Input: part model. Units: mm. Frame: model coordinates. Face numbers are marked on the shaded views. A direction names the side the tool comes from. Round coordinates to 2 decimals unless told otherwise and drop trailing zeros. Loops run counter-clockwise (first coordinate to the right, second up) from the corner with the lowest first, then second, coordinate; pieces in that order, holes last. Notation, with made-up numbers: (-36, -8) -> (-20, -8) arc R22 ccw to (-20, 29) -> close; hole circle Ø9 at (-3, 86.5). An arc over 180 degrees is marked (long way). One line per question, with ' | ' between items. Start each with the question number.
Q1. Mould query, pull axis X, two halves, no side actions, for the marked faces 1, 2 and 3. Classes: pulls with the +X half, pulls with the -X half, needs draft (parallel to the pull), parting line crosses it, or undercut.
Q2. Cut plane D-D on y = 46.5. Return loops of the section in (x, z), and give its area (3 significant figures).
Q3. Access query for the marked faces 4 and 5. Directions: +Z, -Z, +X, -X, +Y, -Y. A direction counts if a zero-diameter tool reaches every point of the face in a straight line with its end or side. Return the directions, or none.
Q4. Material intervals for L1, parallel to Y at x = 0, z = -2.85; L2, parallel to X at y = 46.5, z = -1; L3, parallel to X at y = 5, z = -1, sorted ascending.
Q5. Cut plane B-B on y = 3.5. Return loops of the section in (x, z).
Q6. Contact query for flat-ended pins moving along their axis: P1, Ø4, axis at x = 9, y = 27, coming from the -Z side; P2, Ø2, axis at x = -1.5, y = 22, coming from the -Z side; P3, Ø2, axis at x = -1, z = -3.5, coming from the +Y side; P4, Ø3.5, axis at x = 0, z = -0.5, coming from the -Y side. Output: stop coordinate, or through.
Q7. Cut plane C-C on y = 27. Return loops of the section in (x, z), and give its area (3 significant figures).
Q8. Cut plane A-A on y = 10. Return loops of the section in (x, z), and give its area (3 significant figures).
from build123d import *

# Parameters (mm, degrees)
SKETCH2_W          = 4.5
SKETCH2_H          = 3
CUT_EXTRUDE1_DEPTH = 6
SKETCH3_R          = 1.15
CUT_EXTRUDE2_DEPTH = 6
CUT_EXTRUDE3_DEPTH = 9
SKETCH5_R          = 8
CUT_EXTRUDE4_DEPTH = 5


with BuildPart() as part:
    # Sketch1 → Revolve1 (revolve)
    with BuildSketch(Plane.XY):
        Polygon((0, 50), (-13, 50), (-4, 0), (0, 0), align=None)
    revolve(axis=Axis((0, 0, 0), (0, 1, 0)))

    # Sketch2 → Cut-Extrude1 (cut)
    with BuildSketch(Plane.XZ):
        Rectangle(SKETCH2_W, SKETCH2_H)
    extrude(amount=-CUT_EXTRUDE1_DEPTH, mode=Mode.SUBTRACT)

    # Sketch3 → Cut-Extrude2 (cut)
    with BuildSketch(Plane.XY.offset(-1.5)):
        with Locations((0, 3.5)):
            Circle(SKETCH3_R)
    extrude(amount=-CUT_EXTRUDE2_DEPTH, mode=Mode.SUBTRACT)

    # Sketch4 → Cut-Extrude3 (cut)
    with BuildSketch(Plane(origin=(0, 50, 0), x_dir=(1, 0, 0), z_dir=(0, 1, 0))):
        with BuildLine():
            Line((-8, 0), (-8, -14.002606367))
            Line((-8, -14.002606367), (8, -14.002606367))
            Line((8, -14.002606367), (8, 0))
            ThreePointArc((8, 0), (0, 8), (-8, 0))
        make_face()
    extrude(amount=-CUT_EXTRUDE3_DEPTH, mode=Mode.SUBTRACT)

    # Sketch5 → Cut-Extrude4 (cut)
    with BuildSketch(Plane(origin=(0, 41, 0), x_dir=(1, 0, 0), z_dir=(0, 1, 0))):
        Circle(SKETCH5_R)
    extrude(amount=-CUT_EXTRUDE4_DEPTH, mode=Mode.SUBTRACT)


solid = part.part
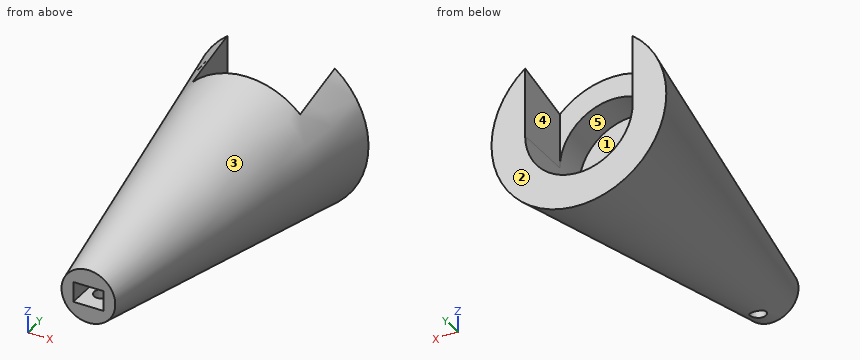
Results:
1) face 1: undercut | face 2: needs draft | face 3: parting line crosses it
2) outline: (-8, 0) -> (-8, 9.43) arc R12.37 ccw (long way) to (8, 9.43) -> (8, 0) arc R8 cw to start | area: 197 mm^2
3) face 4: +Z, +Y | face 5: +Y
4) L1: 0 to 2.35, 4.65 to 36 | L2: -12.33 to -7.94, 7.94 to 12.33 | L3: -4.8 to -2.25, 2.25 to 4.8
5) outline: (-2.25, -1.5) -> (-2.25, 1.5) -> (2.25, 1.5) -> (2.25, -1.5) -> (1.15, -1.5) -> (1.15, -4.48) arc R4.63 ccw (long way) to (-1.15, -4.48) -> (-1.15, -1.5) -> close
6) P1: z = -5.5 | P2: z = -8.05 | P3: y = 36 | P4: y = 0
7) outline: circle Ø17.72 at (0, 0) | area: 247 mm^2
8) outline: circle Ø11.6 at (0, 0) | area: 106 mm^2
